```python
from build123d import *

# Parameters (mm, degrees)
SKETCH1_W           = 23.8
SKETCH1_H           = 11.5
BOSS_EXTRUDE1_DEPTH = 17
SKETCH2_W           = 32.3
SKETCH2_H           = 11.5
BOSS_EXTRUDE2_DEPTH = 2
SKETCH3_R           = 5.75
BOSS_EXTRUDE3_DEPTH = 6
SKETCH4_R           = 2.5
BOSS_EXTRUDE4_DEPTH = 3.2


with BuildPart() as part:
    # Sketch1 → Boss-Extrude1 (new body)
    with BuildSketch(Plane(origin=(0, 0, 0), x_dir=(1, 0, 0), z_dir=(0, 1, 0))):
        with Locations((11.9, 5.75)):
            Rectangle(SKETCH1_W, SKETCH1_H)
    extrude(amount=BOSS_EXTRUDE1_DEPTH)

    # Sketch2 → Boss-Extrude2 (add)
    with BuildSketch(Plane(origin=(0, 17, 0), x_dir=(1, 0, 0), z_dir=(0, 1, 0))):
        with Locations((11.9, 5.75)):
            Rectangle(SKETCH2_W, SKETCH2_H)
    extrude(amount=BOSS_EXTRUDE2_DEPTH)

    # Sketch3 → Boss-Extrude3 (add)
    with BuildSketch(Plane(origin=(0, 19, 0), x_dir=(1, 0, 0), z_dir=(0, 1, 0))):
        with Locations(Location((18.4, 5.75, 0), (0, 0, 270))):
            Circle(SKETCH3_R)
    extrude(amount=BOSS_EXTRUDE3_DEPTH)

    # Sketch4 → Boss-Extrude4 (add)
    with BuildSketch(Plane(origin=(0, 25, 0), x_dir=(1, 0, 0), z_dir=(0, 1, 0))):
        with Locations(Location((18.4, 5.75, 0), (0, 0, 270))):
            Circle(SKETCH4_R)
    extrude(amount=BOSS_EXTRUDE4_DEPTH)


solid = part.part
```
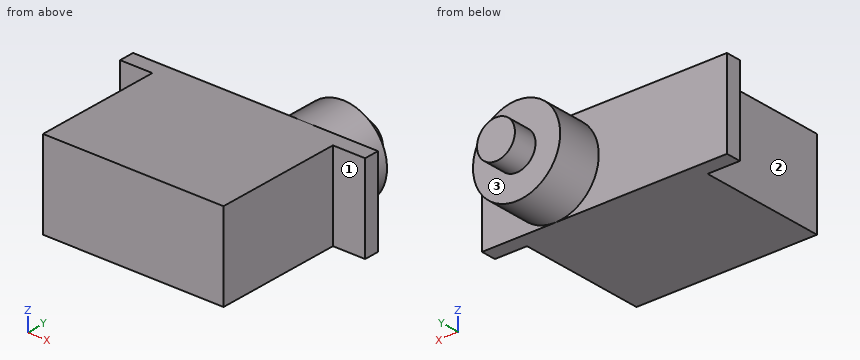
CAD build for the part. Positions are in the model's coordinates, mm. Face numbers are marked on the shaded views. A direction names the side the tool comes from. Coordinates: 2 decimals unless noted, no trailing zeros. Write each loop counter-clockwise with the first axis right and the second up, starting at its lowest first coordinate (ties: lowest second). Pieces come first, ordered by that corner, then holes. Notation, with made-up numbers: (48.5, -20.5) -> (64.5, -20.5) arc R16 ccw to (64.5, -12.5) -> close; hole circle Ø11 at (0, 86). An arc over 180 degrees is marked (long way). Use CSV: the item, a comma, the result in double quotes. Start each with the question number.
Item 1: Tool access for the marked faces 1, 2 and 3: list every direction of +Z, -Z, +X, -X, +Y, -Y with a clear straight run to the whole face (end or side of a thin tool).
Item 2: Band-saw the part on A-A, the plane z = -5.75. Write the cut outline in (x, y).
Item 3: Band-saw the part on D-D, the plane y = 23.25. Write the cut outline in (x, z).
Item 4: Drop flat-ended pins along their axis: P1, Ø4.5, axis at x = -3, z = -8.5, coming from the -Y side; P2, Ø6, axis at x = 10.5, z = -6, coming from the +Y side; P3, Ø2, axis at y = 21, z = -9, coming from the -X side. Give the stop position or say it passes through.
Item 5: Band-saw the part on B-B, the plane x = 13.5. Write the cut outline in (y, z), plus the area to 3 significant figures.
Item 6: Band-saw the part on C-C, the plane y = 5.75. Write the cut outline in (x, z), plus the area to 3 significant figures.
Item 7: Wall check: probe 1 along Y at (x, z) = (8, -4); probe 2 along X at (y, z) = (10.5, -2.25); probe 3 along X at (y, z) = (23.5, -5.75). Give the ranges that are in metal, low to high.
Response values:
1,face 1,"+Z, -Z, +X, -Y"
1,face 2,"+Z, -Z, -X, -Y"
1,face 3,"+Y"
2,outline,"(-4.25, 17) -> (0, 17) -> (0, 0) -> (23.8, 0) -> (23.8, 17) -> (28.05, 17) -> (28.05, 19) -> (24.15, 19) -> (24.15, 25) -> (20.9, 25) -> (20.9, 28.2) -> (15.9, 28.2) -> (15.9, 25) -> (12.65, 25) -> (12.65, 19) -> (-4.25, 19) -> close"
3,outline,"circle Ø11.5 at (18.4, -5.75)"
4,P1,"stops at y = 17"
4,P2,"stops at y = 25"
4,P3,"stops at x = 13.11"
5,outline,"(0, -11.5) -> (19, -11.5) -> (19, -8.76) -> (25, -8.76) -> (25, -2.74) -> (19, -2.74) -> (19, 0) -> (0, 0) -> close"
5,area,"255 mm2"
6,outline,"(0, -11.5) -> (23.8, -11.5) -> (23.8, 0) -> (0, 0) -> close"
6,area,"274 mm2"
7,probe 1,"y = 0 to 19"
7,probe 2,"x = 0 to 23.8"
7,probe 3,"x = 12.65 to 24.15"
